Geometry check sheet. Reference: the model listing, model coordinates, mm. A direction names the side the tool comes from. Give positions to 0.01 mm unless a question says otherwise; leave off trailing zeros. Loops run counter-clockwise (first coordinate to the right, second up) from the corner with the lowest first, then second, coordinate; pieces in that order, holes last. Notation, with made-up numbers: (86.25, 89) -> (115.25, 89) arc R27 ccw to (115.25, 112) -> close; hole circle Ø1 at (66.25, 30.5). An arc over 180 degrees is marked (long way). Answer as a JSON object with one key per item and string values.
from build123d import *

# Parameters (mm, degrees)
SKETCH1_W           = 50.8
SKETCH1_H           = 25.4
BOSS_EXTRUDE1_DEPTH = 12.7
SKETCH2_R           = 6.35
BOSS_EXTRUDE2_DEPTH = 25.4
SKETCH3_R           = 6.35
BOSS_EXTRUDE3_DEPTH = 12.7


with BuildPart() as part:
    # Sketch1 → Boss-Extrude1 (new body)
    with BuildSketch(Plane(origin=(0, 0, 0), x_dir=(1, 0, 0), z_dir=(0, 1, 0))):
        Rectangle(SKETCH1_W, SKETCH1_H)
    extrude(amount=BOSS_EXTRUDE1_DEPTH)

    # Sketch2 → Boss-Extrude2 (add)
    with BuildSketch(Plane(origin=(0, 12.7, 0), x_dir=(1, 0, 0), z_dir=(0, 1, 0))):
        with Locations((-12.7, 0)):
            Circle(SKETCH2_R)
    extrude(amount=BOSS_EXTRUDE2_DEPTH)

    # Sketch3 → Boss-Extrude3 (add)
    with BuildSketch(Plane(origin=(0, 12.7, 0), x_dir=(1, 0, 0), z_dir=(0, 1, 0))):
        with Locations((12.7, 0)):
            Circle(SKETCH3_R)
    extrude(amount=BOSS_EXTRUDE3_DEPTH)


solid = part.part
1) Depth check by flat-ended pin: P1, Ø6.5, axis at x = 13, z = 0.5, coming from the +Y side; P2, Ø4, axis at y = 21, z = 1, coming from the -X side; P3, Ø4, axis at x = 16.5, y = 23.5, coming from the -Z side. Enter the tip coordinate at first touch or a pass-through.
Geometry check:
{"P1": "stops at y = 25.4", "P2": "stops at x = -19.05", "P3": "stops at z = -6.09"}
2) Material ranges on line 1 along Y through (x, z) = (-3, -9.25); line 2 along Y through (x, z) = (10, 3.5); line 3 along X through (y, z) = (24.5, -4.25), recorded low to high. Write a range as from..to.
Geometry check:
{"line 1": "y = 0..12.7", "line 2": "y = 0..25.4", "line 3": "x = -17.42..-7.98, 7.98..17.42"}
3) Section check A-A on x = 12.7. Record the cut outline in (y, z), plus the area to 3 significant figures.
Geometry check:
{"outline": "(0, -12.7) -> (12.7, -12.7) -> (12.7, -6.35) -> (25.4, -6.35) -> (25.4, 6.35) -> (12.7, 6.35) -> (12.7, 12.7) -> (0, 12.7) -> close", "area": "484 mm2"}
4) Section check B-B on z = 0. Record the cut outline in (x, y), plus the area to 3 significant figures.
Geometry check:
{"outline": "(-25.4, 0) -> (25.4, 0) -> (25.4, 12.7) -> (19.05, 12.7) -> (19.05, 25.4) -> (6.35, 25.4) -> (6.35, 12.7) -> (-6.35, 12.7) -> (-6.35, 38.1) -> (-19.05, 38.1) -> (-19.05, 12.7) -> (-25.4, 12.7) -> close", "area": "1,130 mm2"}
5) Section check D-D on y = 34. Record the cut outline in (x, z).
Geometry check:
{"outline": "circle Ø12.7 at (-12.7, 0)"}
6) Section check C-C on y = 15. Record the cut outline in (x, z).
Geometry check:
{"outline": "circle Ø12.7 at (-12.7, 0); circle Ø12.7 at (12.7, 0)"}
7) Tool access check on faces 5 (the face through (6.356, 18.961, -0.279)), 6 (the face through (13, 25.4, 0)), 7 (the face through (0, 6, -12.7)). Record the directions out of +Z, -Z, +X, -X, +Y, -Y that give a thin tool (end or side, any length) a straight path to the whole face; none if there is none.
Geometry check:
{"face 5": "+Y", "face 6": "+Z, -Z, +X, +Y", "face 7": "-Z, +X, -X, +Y, -Y"}
8) Draft check along X on faces 1 (the face through (-13, 38.1, 0)), 2 (the face through (0, 12.7, 0)), 3 (the face through (-25.4, 6, 0)), 4 (the face through (-6.643, 25.222, -1.907)). Enter one of: pulls with the +X half, pulls with the -X half, needs draft (parallel to the pull), parting line crosses it, or undercut.
Geometry check:
{"face 1": "needs draft", "face 2": "undercut", "face 3": "pulls with the -X half", "face 4": "undercut"}
